```python
from build123d import *

# Parameters (mm, degrees)
BOSS_EXTRUDE1_DEPTH = 1.6
SKETCH2_R           = 0.852453889
SKETCH2_R_2         = 0.85
CUT_EXTRUDE1_DEPTH  = 3


with BuildPart() as part:
    # Sketch1 → Boss-Extrude1 (new body)
    with BuildSketch(Plane.XY):
        with BuildLine():
            Line((10.075, 5), (-10.075, 5))
            Line((-10.075, 5), (-10.075, -13.15))
            Line((-10.075, -13.15), (-5.075, -13.15))
            Line((-5.075, -13.15), (-5.075, -5.075))
            ThreePointArc((-5.075, -5.075), (0, 0), (5.075, -5.075))
            Line((5.075, -5.075), (5.075, -13.15))
            Line((5.075, -13.15), (10.075, -13.15))
            Line((10.075, -13.15), (10.075, 5))
        make_face()
    extrude(amount=BOSS_EXTRUDE1_DEPTH)

    # Sketch2 → Cut-Extrude1 (cut)
    with BuildSketch(Plane.XY.offset(1.6)):
        with Locations((5.634338394, 1.936419455)):
            Circle(SKETCH2_R)
        with Locations((-7.907828008, -4.242394056)):
            Circle(SKETCH2_R_2)
    extrude(amount=-CUT_EXTRUDE1_DEPTH, mode=Mode.SUBTRACT)


solid = part.part
```
Source: CAD feature listing. Evaluate the final solid. Frame: model axes, mm. A direction names the side the tool comes from. Give positions to 0.01 mm unless a question says otherwise; leave off trailing zeros. Write each loop counter-clockwise with the first axis right and the second up, starting at its lowest first coordinate (ties: lowest second). Pieces come first, ordered by that corner, then holes.
1. Section query A-A (y = -7.5). Return the cut outline in (x, z) (3 decimals), then the cut area to 3 significant figures.
2. Section query D-D (y = 1.5). Return the cut outline in (x, z) (3 decimals).
3. Section query C-C (x = 3.5). Return the cut outline in (y, z), then the cut area to 3 significant figures.
4. First-contact query: pin 1 (1.5 mm diameter, centred on x = 5.63, y = 1.94, fed in from +Z). Flat tip, straight axial feed; report the tip coordinate or a pass-through.
5. Section query B-B (z = 1.05). Return the cut outline in (x, y) (3 decimals).
6. Access query for faces 5 (the face through (5.075, -9, 1)), 6 (the face through (-8.757, -4.205, 0.811)). Directions: +Z, -Z, +X, -X, +Y, -Y. A direction counts if a zero-diameter tool reaches every point of the face in a straight line with its end or side. Return the directions, or none.
7. Material intervals for line 1 along X through (y, z) = (-9.5, 1.3) (3 decimals); line 2 along Y through (x, z) = (-7.25, 1.2); line 3 along Y through (x, z) = (-8.5, 0.7), sorted ascending.
8. Pull-direction query (Y, two-part tool) for faces 1 (the face through (-8, -13.15, 1)), 2 (the face through (-5.075, -9, 1)), 3 (the face through (0, 5, 1)), 4 (the face through (6.45, 2.19, 0.81)); classes: +Y half, -Y half, draft (parallel to the pull), parting line (faces both ways), or undercut.
Output values:
1. outline: (-10.075, 0) - (-5.075, 0) - (-5.075, 1.6) - (-10.075, 1.6) - close; (5.075, 0) - (10.075, 0) - (10.075, 1.6) - (5.075, 1.6) - close
1. area: 16.0 mm2
2. outline: (-10.075, 0) - (4.902, 0) - (4.902, 1.6) - (-10.075, 1.6) - close; (6.367, 0) - (10.075, 0) - (10.075, 1.6) - (6.367, 1.6) - close
3. outline: (-1.4, 0) - (5, 0) - (5, 1.6) - (-1.4, 1.6) - close
3. area: 10.2 mm2
4. pin 1: passes through
5. outline: (-10.075, -13.15) - (-5.075, -13.15) - (-5.075, -5.075) arc R5.075 cw to (5.075, -5.075) - (5.075, -13.15) - (10.075, -13.15) - (10.075, 5) - (-10.075, 5) - close; hole circle Ø1.7 at (-7.908, -4.242); hole circle Ø1.705 at (5.634, 1.936)
6. face 5: +Z, -Z, -Y
6. face 6: +Z, -Z
7. line 1: x = -10.075 to -5.075, 5.075 to 10.075
7. line 2: y = -13.15 to -4.78, -3.7 to 5
7. line 3: y = -13.15 to -4.85, -3.63 to 5
8. face 1: -Y half
8. face 2: draft
8. face 3: +Y half
8. face 4: undercut
